Here's how the part is built. I have some questions about the finished solid (model axes, mm). A direction names the side the tool comes from. Round coordinates to 2 decimals unless told otherwise and drop trailing zeros. Order: outer loops, then holes, each group sorted by start corner. A loop starts at its lowest first (then second) coordinate and runs counter-clockwise, first axis right, second up. Notation, with made-up numbers: M -2.75,-26.5 L 13.25,-26.5 A16 ccw 13.25,-4.5 Z; hole C 5,10 d10. An arc over 180 degrees is marked long. Answer as CSV lines item,"result". Start each with the question number.
```python
from build123d import *

# Parameters (mm, degrees)
SKETCH1_R           = 2
BOSS_EXTRUDE1_DEPTH = 4
CUT_EXTRUDE1_DEPTH  = 2


with BuildPart() as part:
    # Sketch1 → Boss-Extrude1 (new body)
    with BuildSketch(Plane(origin=(0, 0, 0), x_dir=(1, 0, 0), z_dir=(0, 1, 0))):
        Polygon((-80, 9.45742592), (-65, 24.45742592), (-25, 24.45742592), (25, 24.45742592), (65, 24.45742592), (80, 9.45742592), (80, -10.54257408), (100, -30.54257408), (100, -105.54257408), (80, -125.54257408), (-80, -125.54257408), (-100, -105.54257408), (-100, -30.54257408), (-80, -10.54257408), align=None)
        with Locations(Location((70, -24.316787178, 0), (0, 0, 270))):
            Circle(SKETCH1_R, mode=Mode.SUBTRACT)
        with Locations(Location((-70, -24.316787178, 0), (0, 0, 90))):
            Circle(SKETCH1_R, mode=Mode.SUBTRACT)
        with Locations(Location((70, -95.54257408, 0), (0, 0, 270))):
            Circle(SKETCH1_R, mode=Mode.SUBTRACT)
        with Locations(Location((-70, -95.54257408, 0), (0, 0, 90))):
            Circle(SKETCH1_R, mode=Mode.SUBTRACT)
        with BuildLine():
            Line((10.337598094, -30.54257408), (-10.337598094, -30.54257408))
            ThreePointArc((-10.337598094, -30.54257408), (-17.169948004, -33.372626076), (-20, -40.204975986))
            Line((-20, -40.204975986), (-20, -60.880172175))
            ThreePointArc((-20, -60.880172175), (-17.169948004, -67.712522085), (-10.337598094, -70.54257408))
            Line((-10.337598094, -70.54257408), (10.337598094, -70.54257408))
            ThreePointArc((10.337598094, -70.54257408), (17.169948004, -67.712522085), (20, -60.880172175))
            Line((20, -60.880172175), (20, -40.204975986))
            ThreePointArc((20, -40.204975986), (17.169948004, -33.372626076), (10.337598094, -30.54257408))
        make_face(mode=Mode.SUBTRACT)
    extrude(amount=BOSS_EXTRUDE1_DEPTH)

    # Sketch2 → Cut-Extrude1 (cut)
    # profile 1 of 3: a face of its own
    with BuildSketch(Plane(origin=(0, 4, 0), x_dir=(1, 0, 0), z_dir=(0, 1, 0))):
        Polygon((-25.472812288, -107.11733973), (-18.088196904, -107.11733973), (-18.088196904, -108.348108961), (-24.242043057, -108.348108961), (-24.242043057, -112.040416653), (-18.088196904, -112.040416653), (-18.088196904, -113.271185884), (-24.242043057, -113.271185884), (-24.242043057, -117.886570499), (-18.088196904, -117.886570499), (-18.088196904, -119.11733973), (-25.472812288, -119.11733973), align=None)
    # profile 2 of 3: a face of its own
    with BuildSketch(Plane(origin=(0, 4, 0), x_dir=(1, 0, 0), z_dir=(0, 1, 0))):
        with BuildLine():
            add(Edge.make_bspline(
                [(-2.449254596, -106.809647422), (-2.210250294, -106.815291388), (-1.741137338, -106.826369254), (-1.052600103, -106.910458186), (-0.39562656, -107.057401058), (0.234998612, -107.251617707), (0.833013231, -107.511533008), (1.401913508, -107.825392722), (1.940223039, -108.19794914), (2.443138546, -108.623167189), (2.901482907, -109.087804066), (3.30556983, -109.582626329), (3.641608313, -110.107938076), (3.925601094, -110.655428552), (4.137939972, -111.233761906), (4.293457565, -111.836588501), (4.386018721, -112.46623686), (4.398023561, -112.895080616), (4.404110789, -113.112532038)],
                knots=[0, 0, 0, 0, 1.104339174, 2.167575275, 3.19895946, 4.211974237, 5.212103104, 6.206540156, 7.210035823, 8.232212855, 9.245525355, 10.222267028, 11.178495095, 12.122427609, 13.066774007, 14.018748382, 14.995377748, 16, 16, 16, 16], degree=3))
            add(Edge.make_bspline(
                [(4.404110789, -113.112532038), (4.398050369, -113.328392066), (4.386099229, -113.754067761), (4.293053577, -114.379582401), (4.138376677, -114.979542971), (3.923642546, -115.555449046), (3.645900791, -116.106283535), (3.303525105, -116.630032235), (2.902767408, -117.129340391), (2.445660949, -117.597050461), (1.945808283, -118.023324325), (1.413543804, -118.399049089), (0.854948848, -118.718415341), (0.266006362, -118.975934066), (-0.347638297, -119.179500527), (-0.989897569, -119.319540684), (-1.657446562, -119.409328528), (-2.112422229, -119.419742975), (-2.343485365, -119.425032038)],
                knots=[0, 0, 0, 0, 1.006897034, 1.98559964, 2.943186421, 3.893189035, 4.847917768, 5.815452073, 6.80748931, 7.830684368, 8.862341799, 9.868509738, 10.866468422, 11.859160648, 12.862936224, 13.87796334, 14.922306222, 16, 16, 16, 16], degree=3))
            add(Edge.make_bspline(
                [(-2.343485365, -119.425032038), (-2.576950096, -119.419751502), (-3.036711209, -119.409352567), (-3.71220671, -119.319311427), (-4.360699664, -119.179942779), (-4.980525124, -118.978602698), (-5.5723218, -118.720276019), (-6.137109172, -118.40432461), (-6.672334655, -118.029426015), (-7.173565891, -117.603625551), (-7.631923667, -117.139805588), (-8.034841868, -116.645043071), (-8.372094355, -116.1233088), (-8.651102104, -115.57930445), (-8.869213941, -115.011416487), (-9.022819268, -114.418815701), (-9.116441893, -113.80221707), (-9.128324324, -113.382893249), (-9.13435075, -113.170224345)],
                knots=[0, 0, 0, 0, 1.090007837, 2.146547848, 3.177224824, 4.18441606, 5.184972819, 6.188625542, 7.201944888, 8.232227685, 9.256408654, 10.243626549, 11.2069681, 12.152656664, 13.094449289, 14.042142631, 15.007031417, 16, 16, 16, 16], degree=3))
            add(Edge.make_bspline(
                [(-9.13435075, -113.170224345), (-9.131402402, -113.027503498), (-9.125543406, -112.743886726), (-9.083913012, -112.322131275), (-9.014460276, -111.907586661), (-8.915300454, -111.501446595), (-8.79027069, -111.102737582), (-8.635770803, -110.712430579), (-8.452859537, -110.330424135), (-8.243335129, -109.958340787), (-8.012332045, -109.598947931), (-7.756068538, -109.258983468), (-7.479948492, -108.939194203), (-7.182889634, -108.640362727), (-6.867359525, -108.360919774), (-6.532033375, -108.100372257), (-6.176100518, -107.859172902), (-5.798893902, -107.642516339), (-5.409943928, -107.444915382), (-5.008890938, -107.277563759), (-4.602546124, -107.132145303), (-4.1874152, -107.014075594), (-3.764227753, -106.922537912), (-3.332923423, -106.859004422), (-2.894073915, -106.815043973), (-2.598402752, -106.811456889), (-2.449254596, -106.809647422)],
                knots=[0, 0, 0, 0, 1.000860702, 1.988923732, 2.969140983, 3.946405888, 4.918600368, 5.897447419, 6.887793071, 7.886663957, 8.890501988, 9.881803818, 10.869866848, 11.851371953, 12.834677219, 13.823874237, 14.827633617, 15.847405218, 16.872782081, 17.885187697, 18.892981817, 19.898014594, 20.909858577, 21.927149733, 22.954372848, 24, 24, 24, 24], degree=3))
        make_face()
        with BuildLine():
            add(Edge.make_bspline(
                [(-2.391562288, -108.040416653), (-2.51184609, -108.0418057), (-2.751297347, -108.044570903), (-3.107479041, -108.08096615), (-3.459211644, -108.132822075), (-3.806556963, -108.206786881), (-4.14828776, -108.307535093), (-4.487080949, -108.423686022), (-4.820001205, -108.564158934), (-5.145048651, -108.725339097), (-5.461327271, -108.900684803), (-5.759556253, -109.095930039), (-6.039502965, -109.306760329), (-6.304261521, -109.529097242), (-6.549973838, -109.767761164), (-6.777377431, -110.021526333), (-6.986073395, -110.291257805), (-7.178028363, -110.573366758), (-7.348947973, -110.867432361), (-7.498868436, -111.170494536), (-7.62377932, -111.483313645), (-7.724554049, -111.80421787), (-7.804316815, -112.132626352), (-7.862174528, -112.469031549), (-7.896221771, -112.814553211), (-7.901109212, -113.047553648), (-7.903581519, -113.165416653)],
                knots=[0, 0, 0, 0, 1.034314358, 2.059029303, 3.076765405, 4.092094375, 5.110880351, 6.139806059, 7.171636845, 8.216667878, 9.259764826, 10.280693852, 11.280175756, 12.273075775, 13.252873351, 14.224294354, 15.201858716, 16.184537379, 17.157522275, 18.125488912, 19.09060439, 20.051995777, 21.016643451, 21.995737629, 22.98614617, 24, 24, 24, 24], degree=3))
            add(Edge.make_bspline(
                [(-7.903581519, -113.165416653), (-7.898210266, -113.338737702), (-7.887640897, -113.679793001), (-7.812726489, -114.180904838), (-7.683291296, -114.659574953), (-7.508287161, -115.120354866), (-7.277404332, -115.558281175), (-7.000063223, -115.978132576), (-6.666845655, -116.372061943), (-6.292646829, -116.745390197), (-5.880146385, -117.082729501), (-5.44364821, -117.380106417), (-4.986383542, -117.633010709), (-4.506209078, -117.835958031), (-4.007433542, -117.999585026), (-3.486730857, -118.110234502), (-2.946554931, -118.18376774), (-2.578511943, -118.190727536), (-2.391562288, -118.194262807)],
                knots=[0, 0, 0, 0, 1.001985766, 1.97167371, 2.92126608, 3.864235468, 4.815363556, 5.777764185, 6.767768529, 7.793129838, 8.830022713, 9.843858898, 10.843270901, 11.845781331, 12.853757634, 13.873335827, 14.919748107, 16, 16, 16, 16], degree=3))
            add(Edge.make_bspline(
                [(-2.391562288, -118.194262807), (-2.265694924, -118.192621379), (-2.015966383, -118.189364685), (-1.645104851, -118.157003325), (-1.281395782, -118.104598333), (-0.925240361, -118.029433653), (-0.576244711, -117.935364332), (-0.233153423, -117.823551486), (0.100372074, -117.684715343), (0.427101168, -117.529966058), (0.740175644, -117.354340251), (1.039601812, -117.16560959), (1.318510615, -116.957318496), (1.581165171, -116.736781999), (1.825472925, -116.499862953), (2.050952736, -116.246848151), (2.261725563, -115.980033401), (2.450260234, -115.696029586), (2.621177719, -115.402100516), (2.767700537, -115.097816084), (2.893598008, -114.786452751), (2.997130868, -114.466920991), (3.076803707, -114.139077256), (3.1313758, -113.803085971), (3.16606526, -113.45941233), (3.170902759, -113.22719785), (3.173341558, -113.110128191)],
                knots=[0, 0, 0, 0, 1.078057494, 2.138931934, 3.186396846, 4.224372019, 5.255081129, 6.281828204, 7.313085757, 8.34778727, 9.37721554, 10.386466275, 11.377698063, 12.356805186, 13.322831121, 14.290221845, 15.258318578, 16.233084811, 17.207971885, 18.168911637, 19.123652981, 20.083145109, 21.043790605, 22.010913397, 22.997212883, 24, 24, 24, 24], degree=3))
            add(Edge.make_bspline(
                [(3.173341558, -113.110128191), (3.17090158, -112.993859656), (3.166061946, -112.763244051), (3.131393694, -112.421962658), (3.076744617, -112.088390211), (2.99751732, -111.763602521), (2.893538851, -111.448182118), (2.767688648, -111.141603013), (2.62108354, -110.842157029), (2.450347273, -110.552897813), (2.260835592, -110.2736522), (2.051169953, -110.008485876), (1.822036233, -109.758928429), (1.576327544, -109.520966037), (1.3089803, -109.302162037), (1.02661365, -109.09253243), (0.723417639, -108.901791872), (0.404825644, -108.724478005), (0.075233739, -108.564179625), (-0.261824464, -108.424238717), (-0.604923371, -108.306558799), (-0.951912321, -108.207281647), (-1.305443018, -108.132458501), (-1.662879889, -108.081207676), (-2.025417117, -108.044452246), (-2.268872505, -108.04176892), (-2.391562288, -108.040416653)],
                knots=[0, 0, 0, 0, 0.999618921, 1.982718035, 2.946629433, 3.904142108, 4.854089328, 5.799603779, 6.751722253, 7.718313886, 8.685273778, 9.65154614, 10.6220342, 11.596597958, 12.589904812, 13.590354425, 14.618671442, 15.667306976, 16.72423902, 17.768315198, 18.803281207, 19.841475733, 20.86981583, 21.90753015, 22.945496034, 24, 24, 24, 24], degree=3))
        make_face(mode=Mode.SUBTRACT)
    # profile 3 of 3: a face of its own
    with BuildSketch(Plane(origin=(0, 4, 0), x_dir=(1, 0, 0), z_dir=(0, 1, 0))):
        Polygon((12.896418481, -108.348108961), (12.896418481, -107.11733973), (19.973341558, -107.11733973), (19.973341558, -108.348108961), (17.050264635, -108.348108961), (17.050264635, -119.11733973), (15.819495404, -119.11733973), (15.819495404, -108.348108961), align=None)
    extrude(amount=-CUT_EXTRUDE1_DEPTH, mode=Mode.SUBTRACT)


solid = part.part
```
Item 1: Which directions (+Z, -Z, +X, -X, +Y, -Y) give clear straight access to the entire face, cutting with the end or side of a thin tool? Please do faces 1 (the flat face through (1, 2, -24.457)), 2 (the cylindrical face through (-17.094, 1.972, 33.298)).
Item 2: If we section it at C-C on x = -86: Please give me the cut outline in (y, z).
Item 3: If we section it at A-A on z = 58: Please give me the cut outline in (x, y), and give its area (3 significant figures).
Item 4: If I drill on line 1 along Z through (x, y) = (-70, 2.75); line 2 along X through (y, z) = (3.1, 47.5); line 3 along Z through (x, y) = (67, 2.5), over which ranges is the centre line in solid material (lowest first)?
Item 5: If we section it at B-B on y = 0.85: Please give me the cut outline in (x, z).
Item 6: For P1, Ø6.5, axis at x = -70, z = 24.32, coming from the -Y side; P2, Ø0.6, axis at y = 3.5, z = 112.5, coming from the -X side, each with a flat end and sliding along its axis, tell me the tip position at first contact or that it passes through.
Item 7: If we section it at D-D on z = 17.5: Please give me the cut outline in (x, y).
Item 8: We'd pull the mould along Z, two halves only. Please class faces 3 (the cylindrical face through (17.09, 1.97, 67.79)), 4 (the flat face through (100, 2, 68)), 5 (the flat face through (90.14, 1.97, 115.4)), 6 (the flat face through (-72.605, 1.972, -16.852)): pulls with the +Z half, pulls with the -Z half, needs draft (parallel to the pull), parting line crosses it, or undercut.
Geometry says:
1,face 1,"-Z, +X, -X, +Y, -Y"
1,face 2,"+Y, -Y"
2,outline,"M 0,16.54 L 4,16.54 L 4,119.54 L 0,119.54 Z"
3,outline,"M -100,0 L -20,0 L -20,4 L -100,4 Z; M 20,0 L 100,0 L 100,4 L 20,4 Z"
3,area,"640 mm²"
4,line 1,"-19.46 to 22.32, 26.32 to 93.54, 97.54 to 125.54"
4,line 2,"-100 to -20, 20 to 100"
4,line 3,"-22.46 to 125.54"
5,outline,"M -100,30.54 L -80,10.54 L -80,-9.46 L -65,-24.46 L 65,-24.46 L 80,-9.46 L 80,10.54 L 100,30.54 L 100,105.54 L 80,125.54 L -80,125.54 L -100,105.54 Z; hole C -70,24.32 d4; hole C -70,95.54 d4; hole M -20,40.2 A9.66 ccw -10.34,30.54 L 10.34,30.54 A9.66 ccw 20,40.2 L 20,60.88 A9.66 ccw 10.34,70.54 L -10.34,70.54 A9.66 ccw -20,60.88 Z; hole C 70,24.32 d4; hole C 70,95.54 d4"
6,P1,"y = 0"
6,P2,"x = -93.34"
7,outline,"M -86.96,0 L 86.96,0 L 86.96,4 L -86.96,4 Z"
8,face 3,"undercut"
8,face 4,"needs draft"
8,face 5,"pulls with the +Z half"
8,face 6,"pulls with the -Z half"
